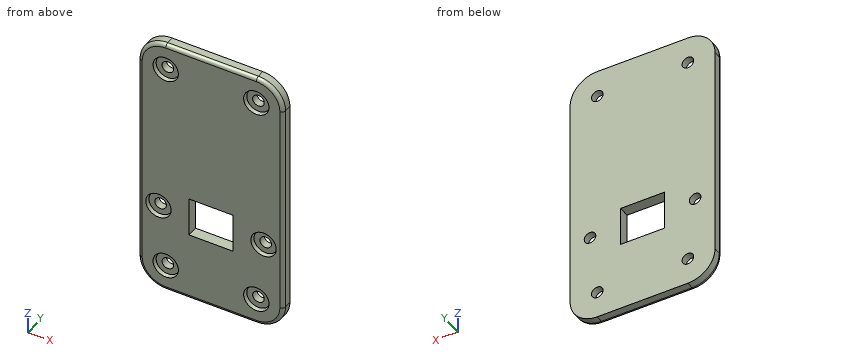
```python
from build123d import *

# Parameters (mm, degrees)
F0_W     = 40
F0_H     = 75
F0_R     = 1.6
F0_W_2   = 12.1
F0_H_2   = 11
F1_DEPTH = 3
F2_R     = 7.5
F3_R     = 3.5
F4_DEPTH = 1
F4_TAPER = 15
F5_R     = 1


with BuildPart() as f1:
    # F0 (on Front) → F1 (new body)
    with BuildSketch(Plane.XZ):
        with Locations((20, 37.5)):
            Rectangle(F0_W, F0_H)
        with Locations((7.5, 7.5)):
            Circle(F0_R, mode=Mode.SUBTRACT)
        with Locations((5.5, 25)):
            Circle(F0_R, mode=Mode.SUBTRACT)
        with Locations((32.5, 7.5)):
            Circle(F0_R, mode=Mode.SUBTRACT)
        with Locations((20, 25)):
            Rectangle(F0_W_2, F0_H_2, mode=Mode.SUBTRACT)
        with Locations((34.5, 25)):
            Circle(F0_R, mode=Mode.SUBTRACT)
        with Locations((7.5, 67.5)):
            Circle(F0_R, mode=Mode.SUBTRACT)
        with Locations((32.5, 67.5)):
            Circle(F0_R, mode=Mode.SUBTRACT)
    extrude(amount=F1_DEPTH)

    # F2
    f2_edges = [f1.edges().sort_by_distance(p)[0] for p in [
        (40, -1.5, 75),
        (40, -1.5, 0),
        (0, -1.5, 0),
        (0, -1.5, 75),
    ]]
    fillet(f2_edges, radius=F2_R)

    # F3 (on face) → F4 (cut)
    with BuildSketch(Plane.XZ.offset(3)):
        with Locations((7.5, 67.5)):
            Circle(F3_R)
        with Locations((32.5, 67.5)):
            Circle(F3_R)
        with Locations((5.5, 25)):
            Circle(F3_R)
        with Locations((32.5, 7.5)):
            Circle(F3_R)
        with Locations((7.5, 7.5)):
            Circle(F3_R)
        with Locations((34.5, 25)):
            Circle(F3_R)
    extrude(amount=-F4_DEPTH, taper=F4_TAPER, mode=Mode.SUBTRACT)

    # F5
    f5_edges = [f1.edges().sort_by_distance(p)[0] for p in [
        (20, -3, 0),
    ]]
    fillet(f5_edges, radius=F5_R)


solid = f1.part
```
Check sheet for the modelled part. Datum: model origin and axes. Units: mm. Round coordinates to 2 decimals unless told otherwise and drop trailing zeros.
1) Section check A-A (z = 25). Give the number of separate pieces and of enclosed holes in the cut face, and give its area (3 significant figures).
2) Go/stop test with flat-tipped pins: pin 1 Ø1.5 at (x, z) = (27.5, 11.5) entering from +Y; pin 2 Ø4 at (x, z) = (7.5, 7.5) entering from -Y. Record where each tip stops, or that it passes through.
3) Scan lines: line 1 (X direction, y = -0.6, z = 7.5); line 2 (Z direction, x = 7.5, y = -1.2); line 3 (X direction, y = -0.7, z = 25). Record each from-to range of solid material in increasing order.
Result:
1. separate pieces: 4
1. enclosed holes: 0
1. area: 57.0 mm2
2. pin 1: stops at y = 0
2. pin 2: stops at y = -2
3. line 1: x = 0 to 5.9, 9.1 to 30.9, 34.1 to 40
3. line 2: z = 0 to 5.9, 9.1 to 65.9, 69.1 to 75
3. line 3: x = 0 to 3.9, 7.1 to 13.95, 26.05 to 32.9, 36.1 to 40
